Design review of the part shown in the three views and the two pictorial views. Dimensions are in mm from the part's minimum x, y and z. Round coordinates to 2 decimals unless told otherwise and drop trailing zeros. Order: outer loops, then holes, each group sorted by start corner. A loop starts at its lowest first (then second) coordinate and runs counter-clockwise, first axis right, second up. Notation, with made-up numbers: (-26.75, 58) - (8.25, 58) arc R20 ccw to (8.25, 63) - close; hole circle Ø1 at (-14, -18). An arc over 180 degrees is marked (long way). One line per item, written item: value.
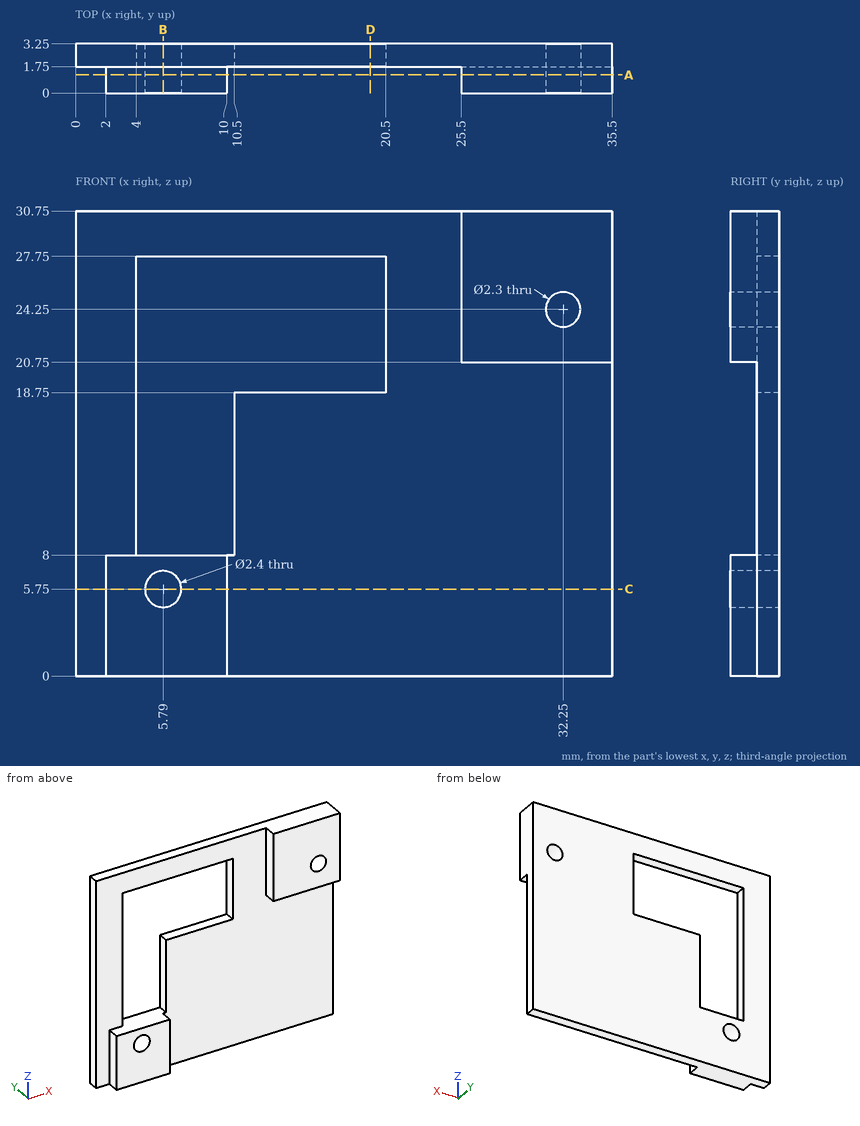
Item 1: Take a section at D-D (x = 19.5). Write out the cut boundary in (y, z), plus the area to 3 significant figures.
Returned:
outline: (1.75, 0) - (3.25, 0) - (3.25, 18.75) - (1.75, 18.75) - close; (1.75, 27.75) - (3.25, 27.75) - (3.25, 30.75) - (1.75, 30.75) - close
area: 32.6 mm^2
Item 2: Take a section at B-B (x = 5.79). Write out the cut boundary in (y, z).
Returned:
outline: (0, 0) - (3.25, 0) - (3.25, 4.55) - (0, 4.55) - close; (0, 6.95) - (3.25, 6.95) - (3.25, 8) - (0, 8) - close; (1.75, 27.75) - (3.25, 27.75) - (3.25, 30.75) - (1.75, 30.75) - close
Item 3: Take a section at A-A (y = 1.2). Write out the cut boundary in (x, z), plus the area to 3 significant figures.
Returned:
outline: (2, 0) - (10, 0) - (10, 8) - (2, 8) - close; (25.5, 20.75) - (35.5, 20.75) - (35.5, 30.75) - (25.5, 30.75) - close; hole circle Ø2.4 at (5.79, 5.75); hole circle Ø2.3 at (32.25, 24.25)
area: 155 mm^2
Item 4: Wall thickness on line 1 (Z direction, x = 32.25, y = 2); line 2 (X direction, y = 1.45, z = 24.25); line 3 (X direction, y = 1.35, z = 5.75): over which ranges is each line inside the solid? List them lowest first.
Returned:
line 1: 0 to 23.1, 25.4 to 30.75
line 2: 25.5 to 31.1, 33.4 to 35.5
line 3: 2 to 4.59, 6.99 to 10
Item 5: Take a section at C-C (z = 5.75). Write out the cut boundary in (x, y), plus the area to 4 significant figures.
Returned:
outline: (0, 1.75) - (2, 1.75) - (2, 0) - (4.59, 0) - (4.59, 3.25) - (0, 3.25) - close; (6.99, 0) - (10, 0) - (10, 1.75) - (35.5, 1.75) - (35.5, 3.25) - (6.99, 3.25) - close
area: 59.45 mm^2
Item 6: For P1, Ø1, axis at x = 5, y = 1, coming from the +Z side; P2, Ø0.9, axis at x = 33, y = 1, coming from the -Z side; P3, Ø1.5, axis at x = 15.5, z = 8.5, coming from the -Y side, all flat-tipped, find the tip position at first contact; note any pin that passes through.
Returned:
P1: z = 8
P2: z = 20.75
P3: y = 1.75
